```python
from build123d import *

# Parameters (mm, degrees)
BOSS_EXTRUDE1_DEPTH = 3.5
SKETCH2_R           = 1.25
BOSS_EXTRUDE2_DEPTH = 6
SKETCH3_R           = 1.25
BOSS_EXTRUDE3_DEPTH = 6


with BuildPart() as part:
    # Sketch1 → Boss-Extrude1 (new body)
    with BuildSketch(Plane.XY):
        with BuildLine():
            Line((-52.349, 2.5), (52.349, 2.5))
            ThreePointArc((52.349, 2.5), (54.849, 0), (52.349, -2.5))
            Line((52.349, -2.5), (-52.349, -2.5))
            ThreePointArc((-52.349, -2.5), (-54.849, 0), (-52.349, 2.5))
        make_face()
    extrude(amount=BOSS_EXTRUDE1_DEPTH)

    # Sketch2 → Boss-Extrude2 (add)
    with BuildSketch(Plane.XY.offset(3.5)):
        with Locations((52.349, 0)):
            Circle(SKETCH2_R)
    extrude(amount=BOSS_EXTRUDE2_DEPTH)

    # Sketch3 → Boss-Extrude3 (add)
    with BuildSketch(Plane(origin=(0, 0, 0), x_dir=(-1, 0, 0), z_dir=(0, 0, -1))):
        with Locations(Location((52.349, 0, 0), (0, 0, 180))):
            Circle(SKETCH3_R)
    extrude(amount=BOSS_EXTRUDE3_DEPTH)


solid = part.part
```
Can you work these out from the model? Positions are in its coordinate system, mm. A direction names the side the tool comes from. Coordinates: 2 decimals unless noted, no trailing zeros. Order: outer loops, then holes, each group sorted by start corner. A loop starts at its lowest first (then second) coordinate and runs counter-clockwise, first axis right, second up.
1. For faces 1 (the face through (52, 0, 9.5)), 2 (the face through (-53.34, 0.76, -2.96)), 3 (the face through (53.54, 0.38, 6.46)), which set-ups out of +Z, -Z, +X, -X, +Y, -Y let a thin tool reach every point of the face, with its end or its side?
2. If we section it at C-C (x = -23): Please give me the cut outline in (y, z), then the cut area to 3 significant figures.
3. I'm going to push flat-ended pins straight in: pin 1 (1.5 mm diameter, centred on y = 0.5, z = -4.5, fed in from -X); pin 2 (1 mm diameter, centred on x = 20, y = 1, fed in from +Z). Where does each tip first touch, or does it pass through?
4. I need wall thicknesses on line 1 (X direction, y = -0.2, z = -2); line 2 (Z direction, x = 37, y = 1.1); line 3 (X direction, y = 0.3, z = 2). Which ranges of each line are inside material? Lowest first, please.
5. If we section it at B-B (z = 5.75): Please give me the cut outline in (x, y), then the cut area to 3 significant figures.
6. If we section it at A-A (y = 0): Please give me the cut outline in (x, z).
Entries:
1. face 1: +Z, +X, -X, +Y, -Y
1. face 2: -Z
1. face 3: +Z
2. outline: (-2.5, 0) - (2.5, 0) - (2.5, 3.5) - (-2.5, 3.5) - close
2. area: 17.5 mm2
3. pin 1: stops at x = -53.6
3. pin 2: stops at z = 3.5
4. line 1: x = -53.58 to -51.12
4. line 2: z = 0 to 3.5
4. line 3: x = -54.83 to 54.83
5. outline: circle Ø2.5 at (52.35, 0)
5. area: 4.91 mm2
6. outline: (-54.85, 0) - (-53.6, 0) - (-53.6, -6) - (-51.1, -6) - (-51.1, 0) - (54.85, 0) - (54.85, 3.5) - (53.6, 3.5) - (53.6, 9.5) - (51.1, 9.5) - (51.1, 3.5) - (-54.85, 3.5) - close
